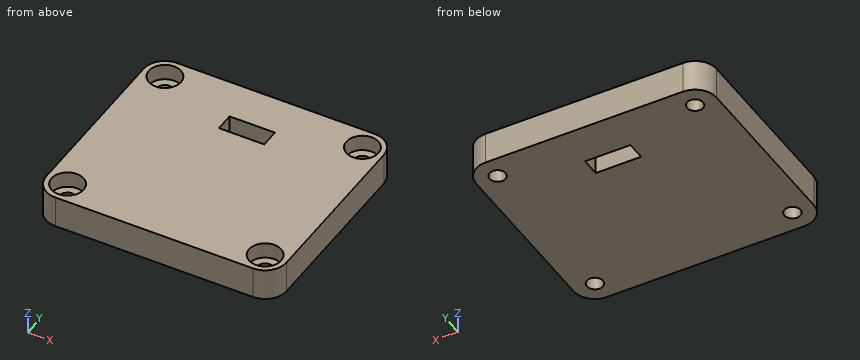
from build123d import *

# Parameters (mm, degrees)
F0_R     = 3
F1_DEPTH = 6
F0_R_2   = 1.5
F2_DEPTH = 3


with BuildPart() as f1:
    # F0 (on Top) → F1 (new body)
    with BuildSketch(Plane.XY):
        with BuildLine():
            ThreePointArc((-20.607047, 18.447905), (-23.435474, 17.276332), (-24.607047, 14.447905))
            Line((-24.607047, 14.447905), (-24.607047, -17.552095))
            ThreePointArc((-24.607047, -17.552095), (-23.435474, -20.380522), (-20.607047, -21.552095))
            Line((-20.607047, -21.552095), (16.392953, -21.552095))
            ThreePointArc((16.392953, -21.552095), (19.22138, -20.380522), (20.392953, -17.552095))
            Line((20.392953, -17.552095), (20.392953, 14.447905))
            ThreePointArc((20.392953, 14.447905), (19.22138, 17.276332), (16.392953, 18.447905))
            Line((16.392953, 18.447905), (-20.607047, 18.447905))
        make_face()
        with Locations((-20.607047, -17.552095)):
            Circle(F0_R, mode=Mode.SUBTRACT)
        with Locations((16.392953, -17.552095)):
            Circle(F0_R, mode=Mode.SUBTRACT)
        Polygon((-14.357047, -13.802095), (-14.357047, 10.697905), (-6.357047, 10.697905), (2.142953, 10.697905), (10.142953, 10.697905), (10.142953, -13.802095), align=None, mode=Mode.SUBTRACT)
        with Locations((-20.607047, 14.447905)):
            Circle(F0_R, mode=Mode.SUBTRACT)
        with Locations((16.392953, 14.447905)):
            Circle(F0_R, mode=Mode.SUBTRACT)
        Polygon((-6.357047, 10.697905), (-14.357047, 10.697905), (-14.357047, -13.802095), (10.142953, -13.802095), (10.142953, 10.697905), (2.142953, 10.697905), (2.142953, 7.197905), (-6.357047, 7.197905), align=None)
    extrude(amount=F1_DEPTH)

    # F0 (on Top) → F2 (join)
    with BuildSketch(Plane.XY):
        with Locations((-20.607047, 14.447905)):
            Circle(F0_R)
        with Locations((-20.607047, 14.447905)):
            Circle(F0_R_2, mode=Mode.SUBTRACT)
        with Locations((16.392953, 14.447905)):
            Circle(F0_R)
        with Locations((16.392953, 14.447905)):
            Circle(F0_R_2, mode=Mode.SUBTRACT)
        with Locations((16.392953, -17.552095)):
            Circle(F0_R)
        with Locations((16.392953, -17.552095)):
            Circle(F0_R_2, mode=Mode.SUBTRACT)
        with Locations((-20.607047, -17.552095)):
            Circle(F0_R)
        with Locations((-20.607047, -17.552095)):
            Circle(F0_R_2, mode=Mode.SUBTRACT)
    extrude(amount=F2_DEPTH)


solid = f1.part
Source: CAD feature listing. Evaluate the final solid. Frame: model axes, mm. Round coordinates to 2 decimals unless told otherwise and drop trailing zeros. Loops run counter-clockwise (first coordinate to the right, second up) from the corner with the lowest first, then second, coordinate; pieces in that order, holes last. Notation, with made-up numbers: (18.25, 68.25) -> (67.25, 68.25) arc R23 cw to (67.25, 107.25) -> close; hole circle Ø6 at (80, 22.25). An arc over 180 degrees is marked (long way). Answer as a JSON object with one key per item and string values. Group by question number.
Q1. Ray query, line 1 (Y direction, x = -20.5, z = 2.5); line 2 (X direction, y = 14.5, z = 3.95); line 3 (Y direction, x = 1, z = 4.1). Return the intervals inside material, ascending. Write a range as from..to.
Q2. Contact query for flat-ended pins moving along their axis: P1, Ø4, axis at x = 16.39, y = 14.45, coming from the +Z side; P2, Ø2.5, axis at x = -20.61, y = -17.55, coming from the +Z side. Output: stop coordinate, or through.
Q3. Section query A-A (x = 0). Output: boundary loops of the cut face in (y, z).
Q4. Section query C-C (y = -17). Output: boundary loops of the cut face in (x, z), plus the area to 3 significant figures.
Q5. Section query B-B (z = 4.9). Output: boundary loops of the cut face in (x, y).
Completed:
{
 "1": {"line 1": "-21.55..-19.05, -16.06..12.95, 15.94..18.45", "line 2": "-24.61..-23.61, -17.61..13.39, 19.39..20.39", "line 3": "-21.55..7.2, 10.7..18.45"},
 "2": {"P1": "z = 3", "P2": "through"},
 "3": {"outline": "(-21.55, 0) -> (7.2, 0) -> (7.2, 6) -> (-21.55, 6) -> close; (10.7, 0) -> (18.45, 0) -> (18.45, 6) -> (10.7, 6) -> close"},
 "4": {"outline": "(-24.61, 0) -> (-22, 0) -> (-22, 3) -> (-23.56, 3) -> (-23.56, 6) -> (-24.61, 6) -> close; (-19.21, 0) -> (15, 0) -> (15, 3) -> (13.44, 3) -> (13.44, 6) -> (-17.66, 6) -> (-17.66, 3) -> (-19.21, 3) -> close; (17.79, 0) -> (20.39, 0) -> (20.39, 6) -> (19.34, 6) -> (19.34, 3) -> (17.79, 3) -> close", "area": "218 mm²"},
 "5": {"outline": "(-24.61, -17.55) arc R4 ccw to (-20.61, -21.55) -> (16.39, -21.55) arc R4 ccw to (20.39, -17.55) -> (20.39, 14.45) arc R4 ccw to (16.39, 18.45) -> (-20.61, 18.45) arc R4 ccw to (-24.61, 14.45) -> close; hole circle Ø6 at (-20.61, -17.55); hole circle Ø6 at (-20.61, 14.45); hole (-6.36, 7.2) -> (2.14, 7.2) -> (2.14, 10.7) -> (-6.36, 10.7) -> close; hole circle Ø6 at (16.39, -17.55); hole circle Ø6 at (16.39, 14.45)"}
}
